```python
from build123d import *
from build123d.topology import SkipClean

# Parameters (mm, degrees)
SKETCH1_R           = 2.850000007
SKETCH1_R_2         = 1.725
BOSS_EXTRUDE1_DEPTH = 6
SKETCH7_R           = 11.125
CUT_EXTRUDE4_DEPTH  = 2.5
SKETCH8_R           = 7.5
CUT_EXTRUDE5_DEPTH  = 6
SKETCH10_R          = 1.725
BOSS_EXTRUDE4_DEPTH = 21
SKETCH11_W          = 3.38
SKETCH11_H          = 26
CUT_EXTRUDE6_DEPTH  = 40.422308
SKETCH14_R          = 1
CUT_EXTRUDE7_DEPTH  = 70.377273429
CHAMFER1_SIZE       = 3
SKETCH19_R          = 4.9
SKETCH19_R_2        = 1
CUT_EXTRUDE9_DEPTH  = 5
SKETCH20_R          = 2.125
CUT_EXTRUDE10_DEPTH = 3
SKETCH21_R          = 2.875
CUT_EXTRUDE11_DEPTH = 3.5
SKETCH22_R          = 2.25
CUT_EXTRUDE12_DEPTH = 82.036885127
CHAMFER5_SIZE       = 3


with BuildPart() as part:
    # Sketch1 → Boss-Extrude1 (new body)
    with BuildSketch(Plane.XY):
        with BuildLine():
            Line((-44.727938028, 20.301676915), (33.883013294, 20.301676915))
            ThreePointArc((33.883013294, 20.301676915), (36.004333638, 19.422997259), (36.883013294, 17.301676915))
            Line((36.883013294, 17.301676915), (36.883013294, -19.198323085))
            ThreePointArc((36.883013294, -19.198323085), (36.004333638, -21.319643428), (33.883013294, -22.198323085))
            Line((33.883013294, -22.198323085), (-44.727938028, -22.198323085))
            ThreePointArc((-44.727938028, -22.198323085), (-46.849258372, -21.319643428), (-47.727938028, -19.198323085))
            Line((-47.727938028, -19.198323085), (-47.727938028, 17.301676915))
            ThreePointArc((-47.727938028, 17.301676915), (-46.849258372, 19.422997259), (-44.727938028, 20.301676915))
        make_face()
        with Locations((-37.727938028, 11.051676915)):
            Circle(SKETCH1_R, mode=Mode.SUBTRACT)
        with Locations((-37.727938028, -12.948323085)):
            Circle(SKETCH1_R, mode=Mode.SUBTRACT)
        with Locations((-7.616986706, 14.551676915)):
            Circle(SKETCH1_R_2, mode=Mode.SUBTRACT)
        with Locations((-7.616986706, -16.448323085)):
            Circle(SKETCH1_R_2, mode=Mode.SUBTRACT)
        with Locations((23.383013294, -16.448323085)):
            Circle(SKETCH1_R_2, mode=Mode.SUBTRACT)
        with Locations((23.383013294, 14.551676915)):
            Circle(SKETCH1_R_2, mode=Mode.SUBTRACT)
    extrude(amount=BOSS_EXTRUDE1_DEPTH)

    # Sketch7 → Cut-Extrude4 (cut)
    with BuildSketch(Plane(origin=(0, 0, 0), x_dir=(-1, 0, 0), z_dir=(0, 0, -1))):
        with Locations((-7.883013294, -0.948323085)):
            Circle(SKETCH7_R)
    extrude(amount=-CUT_EXTRUDE4_DEPTH, mode=Mode.SUBTRACT)

    # Sketch8 → Cut-Extrude5 (cut)
    with BuildSketch(Plane(origin=(0, 0, 0), x_dir=(-1, 0, 0), z_dir=(0, 0, -1))):
        with Locations((-7.883013294, -0.948323085)):
            Circle(SKETCH8_R)
    extrude(amount=-CUT_EXTRUDE5_DEPTH, mode=Mode.SUBTRACT)

    # Sketch10 → Boss-Extrude4 (add)
    with BuildSketch(Plane.XY.offset(6)):
        with BuildLine():
            Line((-12.039294537, 20.301676915), (33.883013294, 20.301676915))
            ThreePointArc((33.883013294, 20.301676915), (36.004333638, 19.422997259), (36.883013294, 17.301676915))
            Line((36.883013294, 17.301676915), (36.883013294, -19.198323085))
            ThreePointArc((36.883013294, -19.198323085), (36.004333638, -21.319643428), (33.883013294, -22.198323085))
            Line((33.883013294, -22.198323085), (-12.039294537, -22.198323085))
            ThreePointArc((-12.039294537, -22.198323085), (-14.160614881, -21.319643428), (-15.039294537, -19.198323085))
            Line((-15.039294537, -19.198323085), (-15.039294537, -13.698323085))
            ThreePointArc((-15.039294537, -13.698323085), (-14.160614881, -11.577002741), (-12.039294537, -10.698323085))
            Line((-12.039294537, -10.698323085), (25.383013294, -10.698323085))
            Line((25.383013294, -10.698323085), (25.383013294, 8.801676915))
            Line((25.383013294, 8.801676915), (-12.039294537, 8.801676915))
            ThreePointArc((-12.039294537, 8.801676915), (-14.160614881, 9.680356572), (-15.039294537, 11.801676915))
            Line((-15.039294537, 11.801676915), (-15.039294537, 17.301676915))
            ThreePointArc((-15.039294537, 17.301676915), (-14.160614881, 19.422997259), (-12.039294537, 20.301676915))
        make_face()
        with Locations((-7.616986706, 14.551676915)):
            Circle(SKETCH10_R, mode=Mode.SUBTRACT)
        with Locations((23.383013294, 14.551676915)):
            Circle(SKETCH10_R, mode=Mode.SUBTRACT)
        with Locations((-7.616986706, -16.448323085)):
            Circle(SKETCH10_R, mode=Mode.SUBTRACT)
        with Locations((23.383013294, -16.448323085)):
            Circle(SKETCH10_R, mode=Mode.SUBTRACT)
    extrude(amount=BOSS_EXTRUDE4_DEPTH)

    # Sketch11 → Cut-Extrude6 (cut)
    with SkipClean():  # the faces are left unmerged after this step: merging them gives an invalid solid
        with BuildSketch(Plane.ZY.offset(15.039294537)):
            with Locations((13, -0.948323085)):
                Rectangle(SKETCH11_W, SKETCH11_H)
        extrude(amount=-CUT_EXTRUDE6_DEPTH, mode=Mode.SUBTRACT)

    # Sketch14 → Cut-Extrude7 (cut, through all)
    with SkipClean():  # the faces are left unmerged after this step: merging them gives an invalid solid
        with BuildSketch(Plane(origin=(0, 20.301676915, 0), x_dir=(1, 0, 0), z_dir=(0, 1, 0))):
            with Locations(Location((1.683013294, -18.19, 0), (0, 0, 270))):
                Circle(SKETCH14_R)
        extrude(amount=-CUT_EXTRUDE7_DEPTH, mode=Mode.SUBTRACT)

    # Chamfer1
    chamfer1_edges = [part.edges().sort_by_distance(p)[0] for p in [
        (1.683013294, -22.198323085, 17.19),
    ]]
    chamfer(chamfer1_edges, length=CHAMFER1_SIZE)

    # Sketch19 → Cut-Extrude9 (cut)
    with SkipClean():  # the faces are left unmerged after this step: merging them gives an invalid solid
        with BuildSketch(Plane(origin=(0, 20.301676915, 0), x_dir=(1, 0, 0), z_dir=(0, 1, 0))):
            with Locations(Location((1.683013294, -18.19, 0), (0, 0, 270))):
                Circle(SKETCH19_R)
            with Locations(Location((1.683013294, -18.19, 0), (0, 0, 270))):
                Circle(SKETCH19_R_2, mode=Mode.SUBTRACT)
        extrude(amount=-CUT_EXTRUDE9_DEPTH, mode=Mode.SUBTRACT)

    # Sketch20 → Cut-Extrude10 (cut)
    with SkipClean():  # the faces are left unmerged after this step: merging them gives an invalid solid
        with BuildSketch(Plane(origin=(0, 15.301676915, 0), x_dir=(1, 0, 0), z_dir=(0, 1, 0))):
            with Locations(Location((1.683013294, -18.19, 0), (0, 0, 270))):
                Circle(SKETCH20_R)
        extrude(amount=-CUT_EXTRUDE10_DEPTH, mode=Mode.SUBTRACT)

    # Sketch21 → Cut-Extrude11 (cut)
    with SkipClean():  # the faces are left unmerged after this step: merging them gives an invalid solid
        with BuildSketch(Plane.XY.offset(27)):
            with Locations((23.383013294, 14.551676915)):
                Circle(SKETCH21_R)
            with Locations((23.383013294, -16.448323085)):
                Circle(SKETCH21_R)
            with Locations((-7.616986706, -16.448323085)):
                Circle(SKETCH21_R)
            with Locations((-7.616986706, 14.551676915)):
                Circle(SKETCH21_R)
        extrude(amount=-CUT_EXTRUDE11_DEPTH, mode=Mode.SUBTRACT)

    # Sketch22 → Cut-Extrude12 (cut, through all)
    with SkipClean():  # the faces are left unmerged after this step: merging them gives an invalid solid
        with BuildSketch(Plane.ZY.offset(-25.383013294)):
            with Locations(Location((18.19, -0.948323085, 0), (0, 0, 270))):
                Circle(SKETCH22_R)
        extrude(amount=-CUT_EXTRUDE12_DEPTH, mode=Mode.SUBTRACT)

    # Chamfer5
    # the kernel refuses this chamfer: 3 mm, written as the material it takes off along each edge
    with BuildSketch(Plane(origin=(1.683013294, 8.801676915, 18.19), x_dir=(0, 0, 1), z_dir=(-1, 0, 0))) as chamfer5_piece_1:
        Polygon((1 + CHAMFER5_SIZE, 0), (1, CHAMFER5_SIZE), (1, 0), align=None)
    revolve(axis=Axis((1.683013294, 8.801676915, 18.19), (0, 1, 0)), mode=Mode.SUBTRACT)


solid = part.part
```
Model file for the job. Use its own axes, mm. A direction names the side the tool comes from. Coordinates: 2 decimals unless noted, no trailing zeros. Loops run counter-clockwise (first coordinate to the right, second up) from the corner with the lowest first, then second, coordinate; pieces in that order, holes last. Notation, with made-up numbers: (-10, 1) - (5, 1) arc R17 cw to (5, 20) - close; hole circle Ø8 at (-4, 62). An arc over 180 degrees is marked (long way). Write item = value, one per line. Start each with the question number.
Item 1: Pull direction Y, two halves, no side cores. Call faces 6 (the face through (-46.83, -21.34, 2.96)), 7 (the face through (-14.184, 19.4, 16.353)), 8 (the face through (5, -12, 11.31)): +Y half, -Y half, draft (parallel to the pull), parting line (faces both ways), or undercut.
Item 2: Saw through at A-A, the plane y = -5.5. List the corners of the cut face in (x, z), then the cut area to 3 significant figures.
Item 3: Saw through at C-C, the plane y = 0. List the corners of the cut face in (x, z), then the cut area to 3 significant figures.
Item 4: Saw through at D-D, the plane x = -8.5. State how many separate pieces and enclosed holes the cut face has, then the cut area to 3 significant figures.
Item 5: Drop flat-ended pins along their axis: pin 1 Ø2 at (x, z) = (2, 18.5) entering from +Y; pin 2 Ø3 at (y, z) = (13.5, 15) entering from -X; pin 3 Ø6 at (y, z) = (3.5, 19) entering from -X; pin 4 Ø2.5 at (y, z) = (-0.95, 18.19) entering from +X. Give the stop position or say it passes through.
Item 6: Saw through at B-B, the plane z = 12.25. List the corners of the cut face in (x, y) (3 decimals), then the cut area to 3 significant figures.
Item 7: 3-axis set-ups, long thin cutter, end or side, ignore diameter. For faces 1 (the face through (1.244, 11.656, 19.248)), 2 (the face through (-15.039, 15, 16)), 3 (the face through (6, -10.698, 9)), 4 (the face through (1.898, 17.837, 13.295)), 5 (the face through (5, -12, 14.69)): which of +Z, -Z, +X, -X, +Y, -Y reach the whole face in a straight line?
Item 8: Wall check: probe 1 along Y at (x, z) = (-7.5, 15.25); probe 2 along Y at (x, z) = (24.5, 17.5); probe 3 along Z at (x, y) = (-3, 10). Give the ranges that are in metal, low to high. Write a range as [from, to].
Answers:
q1.face_6 = -Y half
q1.face_7 = +Y half
q1.face_8 = undercut
q2.outline = (-47.73, 0) - (-2.27, 0) - (-2.27, 2.5) - (1.92, 2.5) - (1.92, 6) - (-47.73, 6) - close; (13.84, 2.5) - (18.03, 2.5) - (18.03, 0) - (36.88, 0) - (36.88, 27) - (25.38, 27) - (25.38, 6) - (13.84, 6) - close
q2.area = 657 mm2
q3.outline = (-47.73, 0) - (-3.2, 0) - (-3.2, 2.5) - (0.44, 2.5) - (0.44, 6) - (-47.73, 6) - close; (15.32, 2.5) - (18.97, 2.5) - (18.97, 0) - (36.88, 0) - (36.88, 16.15) - (25.38, 16.15) - (25.38, 6) - (15.32, 6) - close; (25.38, 20.23) - (36.88, 20.23) - (36.88, 27) - (25.38, 27) - close
q3.area = 595 mm2
q4.separate_pieces = 3
q4.enclosed_holes = 0
q4.area = 538 mm2
q5.pin_1 = 12.3
q5.pin_2 = -15.04
q5.pin_3 = 25.38
q5.pin_4 = through
q6.outline = (-15.039, -19.198) arc R3 ccw to (-12.039, -22.198) - (33.883, -22.198) arc R3 ccw to (36.883, -19.198) - (36.883, 17.302) arc R3 ccw to (33.883, 20.302) - (-12.039, 20.302) arc R3 ccw to (-15.039, 17.302) - (-15.039, 12.052) - (25.383, 12.052) - (25.383, -13.948) - (-15.039, -13.948) - close; hole circle Ø3.45 at (-7.617, -16.448); hole circle Ø3.45 at (-7.617, 14.552); hole circle Ø3.45 at (23.383, -16.448); hole circle Ø3.45 at (23.383, 14.552)
q6.area = 1,110 mm2
q7.face_1 = none
q7.face_2 = +Z, -X, +Y, -Y
q7.face_3 = +Z, -X
q7.face_4 = +Y
q7.face_5 = -X
q8.probe_1 = [-22.2, -18.17], [-14.73, -10.7], [8.8, 12.83], [16.27, 20.3]
q8.probe_2 = [-22.2, -17.76], [-15.13, -10.7], [8.8, 13.24], [15.87, 20.3]
q8.probe_3 = [0, 11.31], [14.69, 27]
